```python
from build123d import *

# Parameters (mm, degrees)
BASE_EXTRUDE_DEPTH = 3


with BuildPart() as part:
    # Sketch1 → Base-Extrude (new body)
    with BuildSketch(Plane.XY):
        with BuildLine():
            Line((-809.531671811, -111.229676779), (-789.61413801, -92.039559057))
            ThreePointArc((-789.61413801, -92.039559057), (-784.29578657, -90.751569276), (-781.326120484, -95.347748455))
            ThreePointArc((-781.326120484, -95.347748455), (-783.901412566, -110.604895358), (-792.031629072, -123.769706047))
            ThreePointArc((-792.031629072, -123.769706047), (-806.92926697, -126.078902011), (-809.531671811, -111.229676779))
        make_face()
        Polygon((-797.390770347, -116.654380858), (-785.42322433, -100.630091722), (-787.826867701, -98.834959819), (-799.794413717, -114.859248956), align=None, mode=Mode.SUBTRACT)
    extrude(amount=BASE_EXTRUDE_DEPTH)


solid = part.part
```
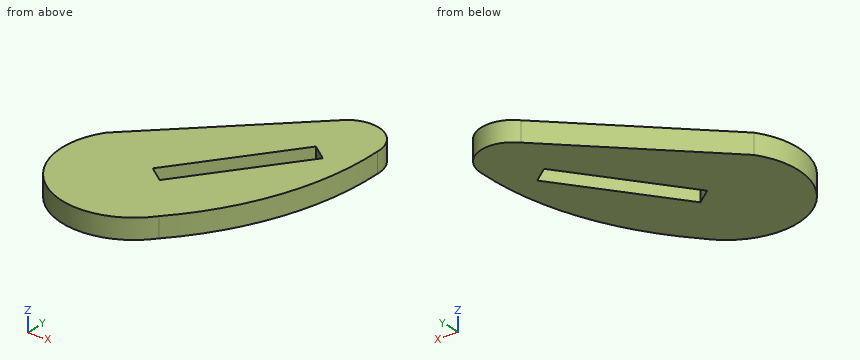
Source: CAD feature listing. Evaluate the final solid. Frame: model axes, mm. Give positions to 0.01 mm unless a question says otherwise; leave off trailing zeros. Write each loop counter-clockwise with the first axis right and the second up, starting at its lowest first coordinate (ties: lowest second). Pieces come first, ordered by that corner, then holes.
1. First-contact query: pin 1 (1 mm diameter, centred on y = -107, z = 1.5, fed in from +X); pin 2 (1.5 mm diameter, centred on y = -100, z = 1.5, fed in from -X). Flat tips, straight axial feed; report the tip coordinate or a pass-through.
2. Section query B-B (z = 2.4). Return the cut outline in (x, y), then the cut area to 3 significant figures.
3. Section query C-C (x = -796.5). Return the cut outline in (y, z), then the cut area to 3 significant figures.
4. Section query A-A (y = -110). Return the cut outline in (x, z), then the cut area to 3 significant figures.
5. Section query D-D (y = -121). Return the cut outline in (x, z).
6. Material intervals for line 1 along X through (y, z) = (-112.5, 0.2); line 2 along X through (y, z) = (-104.5, 1.95); line 3 along Y through (x, z) = (-787, 0.2), sorted ascending.
Output values:
1. pin 1: stops at x = -782.6
1. pin 2: stops at x = -798.65
2. outline: (-809.53, -111.23) arc R10.77 ccw to (-792.03, -123.77) arc R40.33 ccw to (-781.33, -95.35) arc R4.73 ccw to (-789.61, -92.04) - close; hole (-799.79, -114.86) - (-797.39, -116.65) - (-785.42, -100.63) - (-787.83, -98.83) - close
2. area: 627 mm2
3. outline: (-127.26, 0) - (-115.46, 0) - (-115.46, 3) - (-127.26, 3) - close; (-110.45, 0) - (-98.67, 0) - (-98.67, 3) - (-110.45, 3) - close
3. area: 70.7 mm2
4. outline: (-808.26, 0) - (-796.17, 0) - (-796.17, 3) - (-808.26, 3) - close; (-792.42, 0) - (-783.68, 0) - (-783.68, 3) - (-792.42, 3) - close
4. area: 62.5 mm2
5. outline: (-810.78, 0) - (-789.69, 0) - (-789.69, 3) - (-810.78, 3) - close
6. line 1: x = -810.28 to -798.03, -794.29 to -784.67
6. line 2: x = -802.55 to -792.06, -788.31 to -782.14
6. line 3: y = -117.04 to -102.74, -99.45 to -90.51
